Source: three-view drawing plus pictorial views. Frame: mm from the lowest corner of the part. A direction names the side the tool comes from. Give positions to 0.01 mm unless a question says otherwise; leave off trailing zeros. Write each loop counter-clockwise with the first axis right and the second up, starting at its lowest first coordinate (ties: lowest second). Pieces come first, ordered by that corner, then holes.
Q1. Cut plane A-A on y = 6.5. Return the cut outline in (x, z).
Q2. Draft query along X for the marked faces 1, 2, 3 and 4. Return one class per face: pulls with the +X half, pulls with the -X half, needs draft (parallel to the pull), parting line crosses it, or undercut.
Q3. Cut plane D-D on y = 8. Return the cut outline in (x, z).
Q4. Cut plane B-B on x = 5.5. Return the cut outline in (y, z).
Q5. Reachability of the marked faces 5 and 6 from +Z, -Z, +X, -X, +Y, -Y: full face, straight path, thin tool, end or side. Return the list, or none.
Q6. Pin query (flat end, axial travel): pin 1 (1 mm diameter, centred on x = 4.5, z = 5, fed in from +Y); pin 2 (4 mm diameter, centred on y = 9.5, z = 4.5, fed in from -X); pin 3 (4 mm diameter, centred on x = 4.5, z = 2.5, fed in from +Y). Return the tip coordinate at first contact, or that it passes through.
Q7. Line query: L1, parallel to X at y = 12.25, z = 2.25; L2, parallel to Y at x = 6, z = 6.5; L3, parallel to X at y = 0.25, z = 4 (1 decimal). Output: solid intervals per line, ascending.
Q8. Cut plane C-C on z = 4.25. Return the cut outline in (x, y).
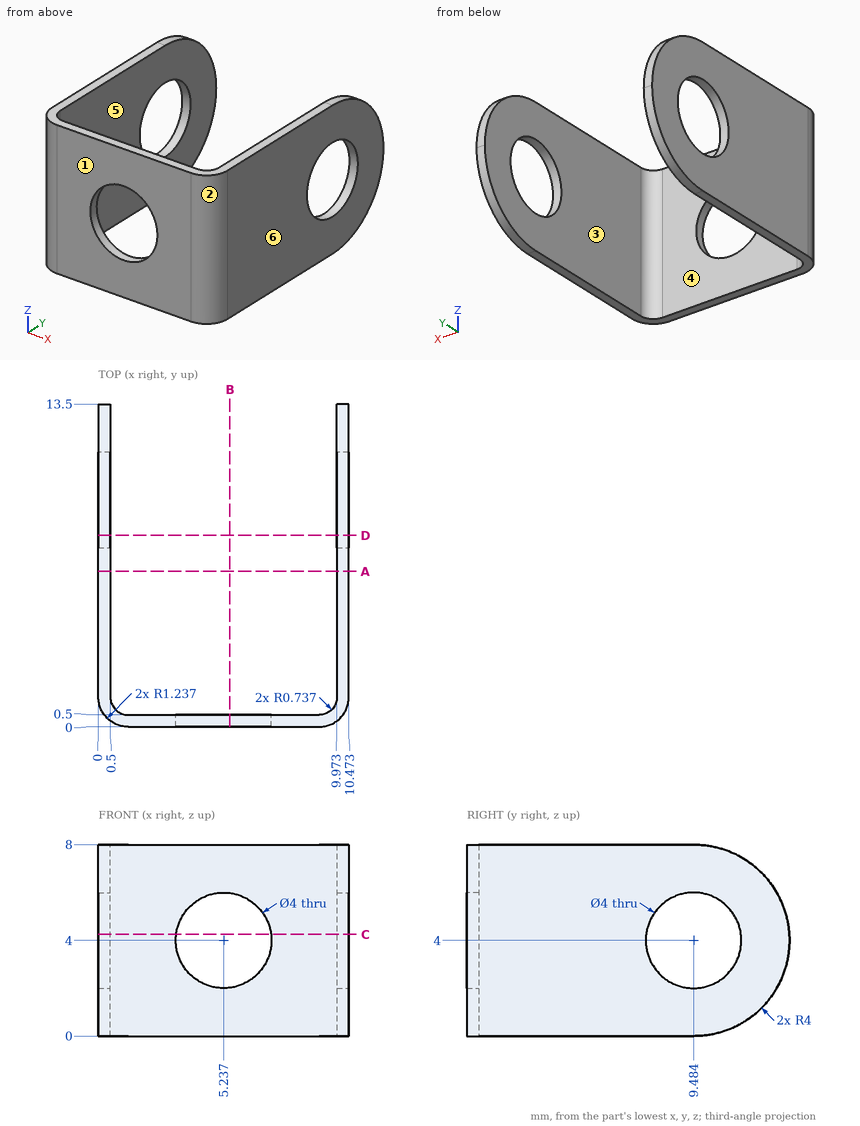
Data:
1. outline: (0, 0) - (0.5, 0) - (0.5, 8) - (0, 8) - close; (9.97, 0) - (10.47, 0) - (10.47, 8) - (9.97, 8) - close
2. face 1: needs draft
2. face 2: pulls with the +X half
2. face 3: undercut
2. face 4: undercut
3. outline: (0, 0) - (0.5, 0) - (0.5, 2.66) - (0, 2.66) - close; (0, 5.34) - (0.5, 5.34) - (0.5, 8) - (0, 8) - close; (9.97, 0) - (10.47, 0) - (10.47, 2.66) - (9.97, 2.66) - close; (9.97, 5.34) - (10.47, 5.34) - (10.47, 8) - (9.97, 8) - close
4. outline: (0, 0) - (0.5, 0) - (0.5, 2.02) - (0, 2.02) - close; (0, 5.98) - (0.5, 5.98) - (0.5, 8) - (0, 8) - close
5. face 5: +Z, -Z, +Y
5. face 6: +Z, -Z, +X, +Y, -Y
6. pin 1: passes through
6. pin 2: stops at x = 0
6. pin 3: stops at y = 0.5
7. L1: x = 0 to 0.5, 9.97 to 10.47
7. L2: y = 0 to 0.5
7. L3: x = 0.5 to 3.2, 7.2 to 10
8. outline: (0, 1.24) arc R1.24 ccw to (1.24, 0) - (3.25, 0) - (3.25, 0.5) - (1.24, 0.5) arc R0.74 cw to (0.5, 1.24) - (0.5, 7.5) - (0, 7.5) - close; (0, 11.47) - (0.5, 11.47) - (0.5, 13.49) - (0, 13.49) - close; (7.22, 0) - (9.24, 0) arc R1.24 ccw to (10.47, 1.24) - (10.47, 7.5) - (9.97, 7.5) - (9.97, 1.24) arc R0.74 cw to (9.24, 0.5) - (7.22, 0.5) - close; (9.97, 11.47) - (10.47, 11.47) - (10.47, 13.49) - (9.97, 13.49) - close
